Read the model definition and answer for the solid it produces. Units are mm, in the model's axes. A direction names the side the tool comes from. Coordinates: 2 decimals unless noted, no trailing zeros. Order: outer loops, then holes, each group sorted by start corner. A loop starts at its lowest first (then second) coordinate and runs counter-clockwise, first axis right, second up. Notation, with made-up numbers: (-28, 0.25) - (-22, 0.25) arc R13 ccw to (-22, 15.25) - close; hole circle Ø8 at (-4, 50). An arc over 180 degrees is marked (long way). Write item = value, one per line.
from build123d import *

# Parameters (mm, degrees)
SKETCH1_R           = 7.5
BOSS_EXTRUDE1_DEPTH = 200
BOSS_EXTRUDE2_START = -100
SKETCH2_R           = 12.5
BOSS_EXTRUDE2_DEPTH = 5


with BuildPart() as part:
    # Sketch1 → Boss-Extrude1 (new body)
    with BuildSketch(Plane(origin=(0, 0, 0), x_dir=(1, 0, 0), z_dir=(0, 1, 0))):
        with Locations(Location((0, 0, 0), (0, 0, 270))):
            Circle(SKETCH1_R)
    extrude(amount=BOSS_EXTRUDE1_DEPTH)

    # Sketch2 → Boss-Extrude2 (add)
    with BuildSketch(Plane(origin=(0, 200, 0), x_dir=(1, 0, 0), z_dir=(0, 1, 0)).offset(BOSS_EXTRUDE2_START)):
        with Locations(Location((0, 0, 0), (0, 0, 270))):
            Circle(SKETCH2_R)
    extrude(amount=BOSS_EXTRUDE2_DEPTH)


solid = part.part
1) The part is cut by section D-D (y = 43.5). Determine the outline of the cut face in (x, z).
Returned:
outline = circle Ø15 at (0, 0)
2) The part is cut by section B-B (z = -3). Determine the outline of the cut face in (x, y), and give its area (3 significant figures).
Returned:
outline = (-12.13, 100) - (-6.87, 100) - (-6.87, 0) - (6.87, 0) - (6.87, 100) - (12.13, 100) - (12.13, 105) - (6.87, 105) - (6.87, 200) - (-6.87, 200) - (-6.87, 105) - (-12.13, 105) - close
area = 2,800 mm^2
3) The part is cut by section A-A (x = 0). Determine the outline of the cut face in (y, z).
Returned:
outline = (0, -7.5) - (100, -7.5) - (100, -12.5) - (105, -12.5) - (105, -7.5) - (200, -7.5) - (200, 7.5) - (105, 7.5) - (105, 12.5) - (100, 12.5) - (100, 7.5) - (0, 7.5) - close
4) For faces 1 (the face through (0, 200, 0)), 2 (the face through (0.33, 151.835, -7.493)), 3 (the face through (-8, 100, 0)), determine the directions among +Z, -Z, +X, -X, +Y, -Y from which every point of the face is accessible in a straight line to the end or side of a thin tool.
Returned:
face_1 = +Z, -Z, +X, -X, +Y
face_2 = +Y
face_3 = -Y
5) The part is cut by section C-C (y = 102.5). Determine the outline of the cut face in (x, z).
Returned:
outline = circle Ø25 at (0, 0)
6) Flat-ended cylindrical pins translate along their axes: pin 1 Ø12.5 at (x, z) = (5, 3) entering from -Y; pin 2 Ø1.5 at (x, z) = (-8.5, 2) entering from -Y; pin 3 Ø2 at (x, z) = (9.5, 4.5) entering from +Y; pin 4 Ø10 at (x, y) = (1.5, 146) entering from -Z. Find the tip coordinate at first contact, or state that the pin passes through.
Returned:
pin_1 = 0
pin_2 = 100
pin_3 = 105
pin_4 = -7.5
7) Straight lines are drawn through the part: line 1 along Y through (x, z) = (6, -6); line 2 along Z through (x, y) = (0.25, 140); line 3 along Z through (x, y) = (-1.75, 102). For each, find the intervals that lie inside material, in ascending order. Write a range as from..to.
Returned:
line_1 = 100..105
line_2 = -7.5..7.5
line_3 = -12.38..12.38
